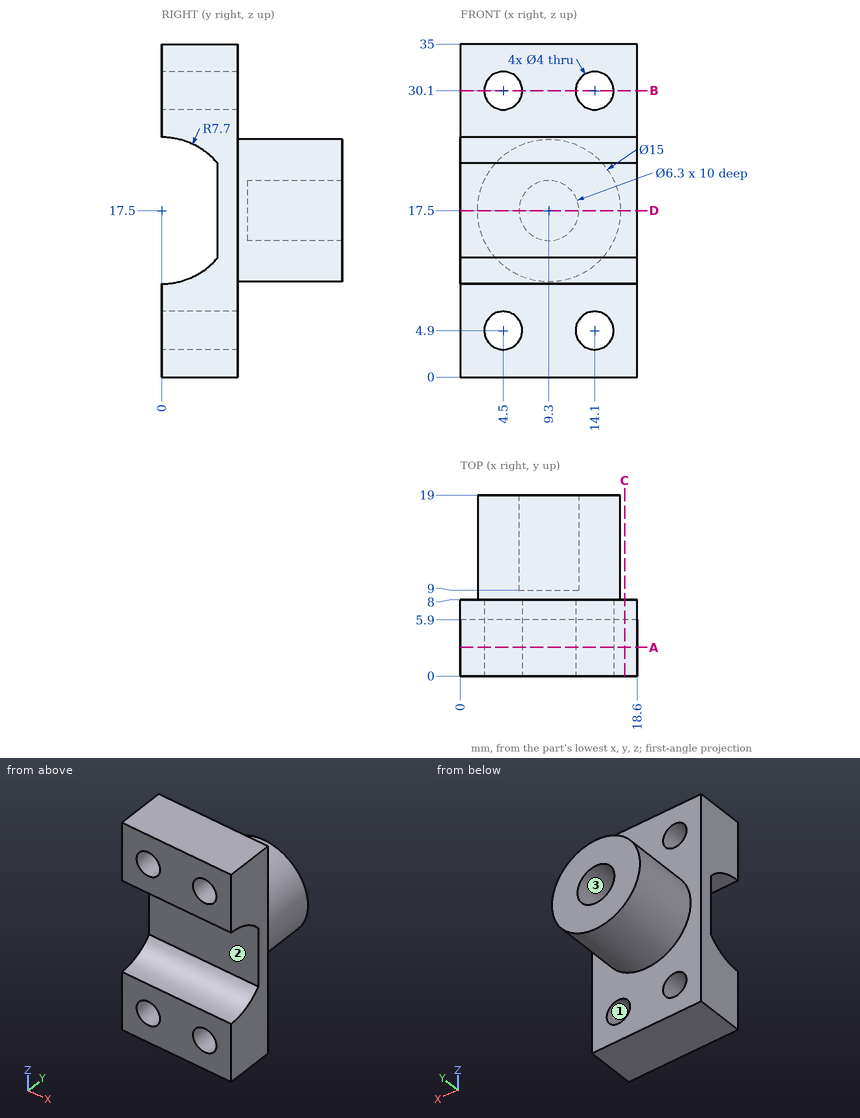
Geometry check sheet. Reference: drawing and pictorial views, mm from the part's lowest x, y, z. A direction names the side the tool comes from. Round coordinates to 2 decimals unless told otherwise and drop trailing zeros. Loops run counter-clockwise (first coordinate to the right, second up) from the corner with the lowest first, then second, coordinate; pieces in that order, holes last. Notation, with made-up numbers: (5.25, 31.5) - (16.25, 31.5) arc R15 cw to (16.25, 37.5) - close; hole circle Ø1 at (61, -37). An arc over 180 degrees is marked (long way). Write item = value, one per line. Start each with the question number.
Q1. Thickness scan on L1, parallel to X at y = 4, z = 30.1; L2, parallel to Z at x = 15.75, y = 1.5; L3, parallel to Z at x = 9.75, y = 1.75. Record the ranges inside material, lowest first.
Q2. Section check C-C (x = 17.25). Record the boundary of the cut face in (y, z).
Q3. Access from +Z, -Z, +X, -X, +Y, -Y to the whole of each face (thin tool, end or side, straight path). Record for the marked faces 1, 2 and 3.
Q4. Section check B-B (z = 30.1). Record the boundary of the cut face in (x, y).
Q5. Depth check by flat-ended pin: P1, Ø2, axis at x = 12, z = 5.5, coming from the +Y side; P2, Ø3, axis at y = 13, z = 11.5, coming from the -X side; P3, Ø5, axis at x = 7, z = 17, coming from the -Y side. Enter the tip coordinate at first touch or a pass-through.
Q6. Section check D-D (z = 17.5). Record the boundary of the cut face in (x, y).
Q7. Section check A-A (y = 3). Record the boundary of the cut face in (x, z), plus the area to 3 significant figures.
Derived:
q1.L1 = 0 to 2.5, 6.5 to 12.1, 16.1 to 18.6
q1.L2 = 0 to 3.77, 6.03 to 9.95, 25.05 to 28.97, 31.23 to 35
q1.L3 = 0 to 10, 25 to 35
q2.outline = (0, 0) - (8, 0) - (8, 35) - (0, 35) - (0, 25.2) arc R7.7 cw to (5.9, 22.45) - (5.9, 12.55) arc R7.7 cw to (0, 9.8) - close
q3.face_1 = +Y, -Y
q3.face_2 = +X, -X, -Y
q3.face_3 = +Y
q4.outline = (0, 0) - (2.5, 0) - (2.5, 8) - (0, 8) - close; (6.5, 0) - (12.1, 0) - (12.1, 8) - (6.5, 8) - close; (16.1, 0) - (18.6, 0) - (18.6, 8) - (16.1, 8) - close
q5.P1 = 8
q5.P2 = 3.3
q5.P3 = 5.9
q6.outline = (0, 5.9) - (18.6, 5.9) - (18.6, 8) - (16.8, 8) - (16.8, 19) - (12.45, 19) - (12.45, 9) - (6.15, 9) - (6.15, 19) - (1.8, 19) - (1.8, 8) - (0, 8) - close
q7.outline = (0, 0) - (18.6, 0) - (18.6, 10.41) - (0, 10.41) - close; (0, 24.59) - (18.6, 24.59) - (18.6, 35) - (0, 35) - close; hole circle Ø4 at (4.5, 4.9); hole circle Ø4 at (4.5, 30.1); hole circle Ø4 at (14.1, 4.9); hole circle Ø4 at (14.1, 30.1)
q7.area = 337 mm^2
